```python
from build123d import *

# Parameters (mm, degrees)
BOSS_EXTRUDE1_DEPTH = 0.91
SKETCH9_R           = 5.15
CUT_EXTRUDE3_DEPTH  = 127.575385048
VISION_PATTERN_R    = 25
VISION_PATTERN_R_2  = 20
CUT_EXTRUDE4_DEPTH  = 127.575385048
FILLET1_R           = 10


with BuildPart() as part:
    # Sketch1 → Boss-Extrude1 (new body)
    with BuildSketch(Plane(origin=(0, 0, 0), x_dir=(1, 0, 0), z_dir=(0, 1, 0))):
        with BuildLine():
            Line((-48.839021284, -75), (48.839021284, -75))
            ThreePointArc((48.839021284, -75), (0, 89.5), (-48.839021284, -75))
        make_face()
    extrude(amount=-BOSS_EXTRUDE1_DEPTH)

    # Sketch9 → Cut-Extrude3 (cut, through all)
    with BuildSketch(Plane(origin=(0, 0, 0), x_dir=(1, 0, 0), z_dir=(0, 1, 0))):
        with Locations(Location((78.541209232, -8.501673503, 0), (0, 0, 270))):
            Circle(SKETCH9_R)
        with Locations(Location((-78.541209232, -8.501673503, 0), (0, 0, 270))):
            Circle(SKETCH9_R)
    extrude(amount=-CUT_EXTRUDE3_DEPTH, mode=Mode.SUBTRACT)

    # Vision Pattern → Cut-Extrude4 (cut, through all)
    with BuildSketch(Plane(origin=(0, 0, 0), x_dir=(1, 0, 0), z_dir=(0, 1, 0))):
        with Locations(Location((0, 0, 0), (0, 0, 270))):
            Circle(VISION_PATTERN_R)
        with Locations(Location((54.772255751, -35, 0), (0, 0, 270))):
            Circle(VISION_PATTERN_R_2)
        with Locations(Location((-54.772255751, -35, 0), (0, 0, 270))):
            Circle(VISION_PATTERN_R_2)
        with Locations(Location((35, 54.772255751, 0), (0, 0, 270))):
            Circle(VISION_PATTERN_R_2)
        with Locations(Location((-35, 54.772255751, 0), (0, 0, 270))):
            Circle(VISION_PATTERN_R_2)
    extrude(amount=-CUT_EXTRUDE4_DEPTH, mode=Mode.SUBTRACT)

    # Fillet1
    fillet1_edges = [part.edges().sort_by_distance(p)[0] for p in [
        (48.839021284, -0.455, 75),
        (-48.839021284, -0.455, 75),
    ]]
    fillet(fillet1_edges, radius=FILLET1_R)


solid = part.part
```
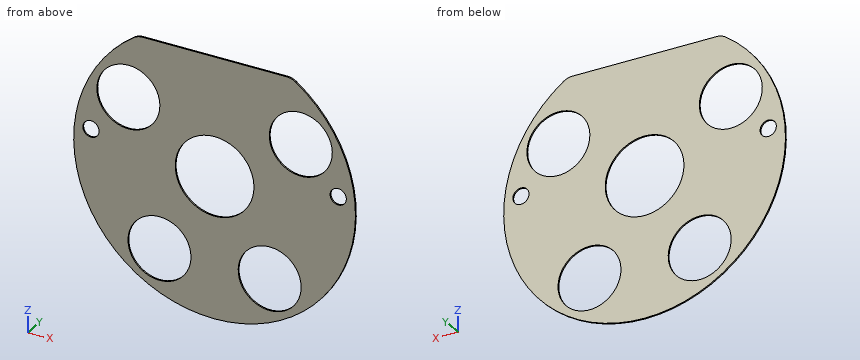
Source: CAD feature listing. Evaluate the final solid. Frame: model axes, mm. Round coordinates to 2 decimals unless told otherwise and drop trailing zeros. Loops run counter-clockwise (first coordinate to the right, second up) from the corner with the lowest first, then second, coordinate; pieces in that order, holes last. Notation, with made-up numbers: M 71.25,54 L 104.25,54 A13 cw 104.25,63 Z; hole C 29,-39 d2. An arc over 180 degrees is marked long. Use a Markdown table: item, result. Add a question column.
1. Cut plane C-C, the plane z = 35. Output: boundary loops of the cut face in (x, y).
2. Ray query, line 1 along Z through (x, y) = (-1, -0.75); line 2 along X through (y, z) = (-0.4, 0); line 3 along Z through (x, y) = (-53.5, -0.15). Return the intervals inside material, ascending. Write a range as [from, to].
3. Cut plane A-A, the plane z = 0. Output: boundary loops of the cut face in (x, y).
4. Cut plane D-D, the plane y = -0.5. Output: boundary loops of the cut face in (x, z).
5. Cut plane B-B, the plane x = 0. Output: boundary loops of the cut face in (y, z).
6. Contact query for flat-ended pins moving along their axis: pin 1 (9.5 mm diameter, centred on x = 78.54, z = 8.5, fed in from -Y); pin 2 (8 mm diameter, centred on x = 13.5, z = 52.5, fed in from +Y). Output: stop coordinate, or through.
Solution:
| question | item | result |
|---|---|---|
| 1 | outline | M -82.37,-0.91 L -74.77,-0.91 L -74.77,0 L -82.37,0 Z; M -34.77,-0.91 L 34.77,-0.91 L 34.77,0 L -34.77,0 Z; M 74.77,-0.91 L 82.37,-0.91 L 82.37,0 L 74.77,0 Z |
| 2 | line 1 | z = [-89.49, -24.98], [24.98, 75] |
| 2 | line 2 | x = [-89.5, -25], [25, 89.5] |
| 2 | line 3 | z = [-71.75, -62.37], [-47.17, 15.04], [54.96, 71.75] |
| 3 | outline | M -89.5,-0.91 L -25,-0.91 L -25,0 L -89.5,0 Z; M 25,-0.91 L 89.5,-0.91 L 89.5,0 L 25,0 Z |
| 4 | outline | M -51.53,73.18 A89.5 ccw long 51.53,73.18 A10 ccw 45.77,75 L -45.77,75 A10 ccw Z; hole C -78.54,8.5 d10.3; hole C -54.77,35 d40; hole C -35,-54.77 d40; hole C 0,0 d50; hole C 35,-54.77 d40; hole C 54.77,35 d40; hole C 78.54,8.5 d10.3 |
| 5 | outline | M -0.91,-89.5 L 0,-89.5 L 0,-25 L -0.91,-25 Z; M -0.91,25 L 0,25 L 0,75 L -0.91,75 Z |
| 6 | pin 1 | passes through |
| 6 | pin 2 | stops at y = 0 |
